Job drawing, mm, ordinate dimensions from the low corner. One solid piece. A direction names the side the tool comes from. Give positions to 0.01 mm unless a question says otherwise; leave off trailing zeros. Loops run counter-clockwise (first coordinate to the right, second up) from the corner with the lowest first, then second, coordinate; pieces in that order, holes last. Notation, with made-up numbers: (-12.75, 24) -> (34.25, 24) arc R6 ccw to (34.25, 35) -> close; hole circle Ø1 at (-36.5, 51.25). An arc over 180 degrees is marked (long way). Use one line per item in the form item = value.
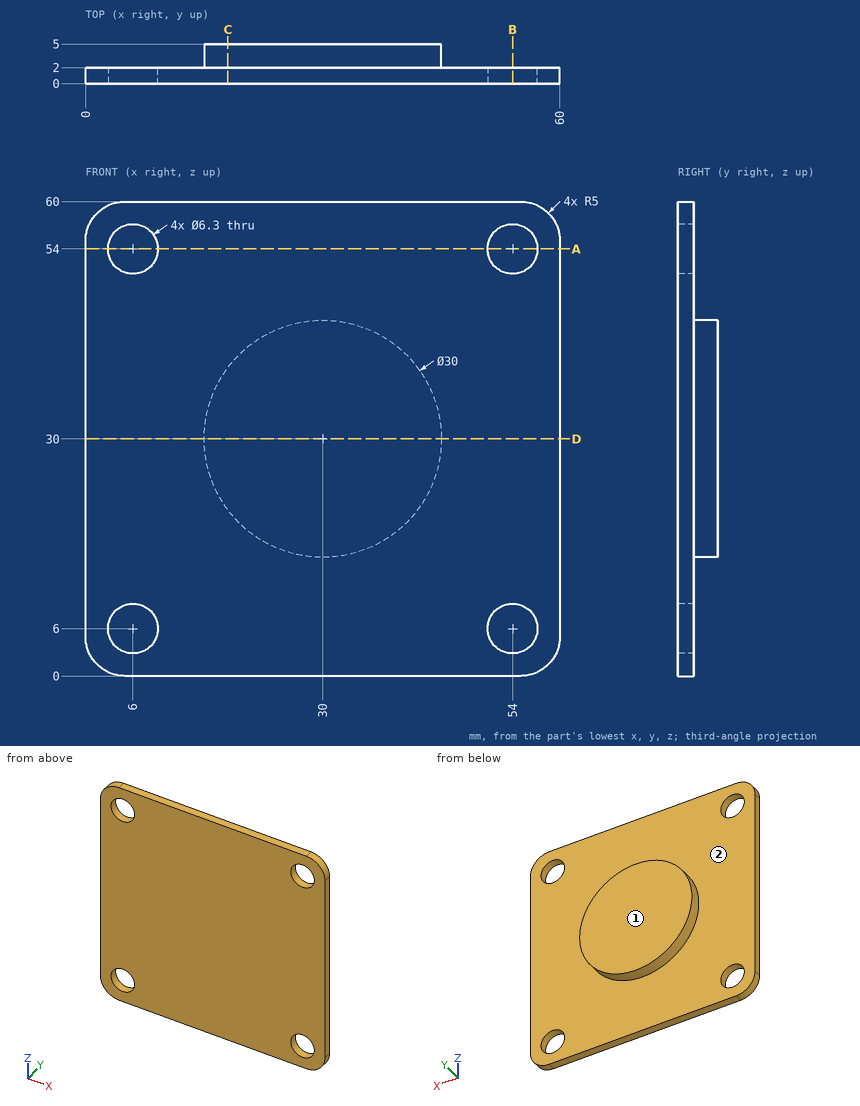
1. Cut at B-B, the plane x = 54. Write the cut outline in (y, z), then the cut area to 3 significant figures.
Result sheet:
outline = (0, 0) -> (2, 0) -> (2, 2.85) -> (0, 2.85) -> close; (0, 9.15) -> (2, 9.15) -> (2, 50.85) -> (0, 50.85) -> close; (0, 57.15) -> (2, 57.15) -> (2, 60) -> (0, 60) -> close
area = 94.8 mm^2
2. Tool access for the marked faces 1 and 2: list every direction of +Z, -Z, +X, -X, +Y, -Y with a clear straight run to the whole face (end or side of a thin tool).
Result sheet:
face_1 = +Z, -Z, +X, -X, +Y
face_2 = +Y
3. Cut at D-D, the plane z = 30. Write the cut outline in (x, y).
Result sheet:
outline = (0, 0) -> (60, 0) -> (60, 2) -> (45, 2) -> (45, 5) -> (15, 5) -> (15, 2) -> (0, 2) -> close
4. Drop flat-ended pins along their axis: P1, Ø5, axis at x = 6, z = 6, coming from the +Y side; P2, Ø4, axis at x = 42, z = 6.5, coming from the +Y side. Give the stop position or say it passes through.
Result sheet:
P1 = through
P2 = 2
5. Cut at C-C, the plane x = 18. Write the cut outline in (y, z).
Result sheet:
outline = (0, 0) -> (2, 0) -> (2, 21) -> (5, 21) -> (5, 39) -> (2, 39) -> (2, 60) -> (0, 60) -> close
6. Drill centre lines: line 1 (X direction, y = 0.7, z = 54); line 2 (Z direction, x = 30.5, y = 2.9). Where is each one in solid material? Low to high.
Result sheet:
line_1 = 0 to 2.85, 9.15 to 50.85, 57.15 to 60
line_2 = 15.01 to 44.99
7. Cut at A-A, the plane z = 54. Write the cut outline in (x, y), then the cut area to 3 significant figures.
Result sheet:
outline = (0, 0) -> (2.85, 0) -> (2.85, 2) -> (0, 2) -> close; (9.15, 0) -> (50.85, 0) -> (50.85, 2) -> (9.15, 2) -> close; (57.15, 0) -> (60, 0) -> (60, 2) -> (57.15, 2) -> close
area = 94.8 mm^2
